Could you check a few things on this drawing? It's one solid part, dimensions in mm from its lowest x, y, z. Coordinates: 2 decimals unless noted, no trailing zeros. Order: outer loops, then holes, each group sorted by start corner. A loop starts at its lowest first (then second) coordinate and runs counter-clockwise, first axis right, second up.
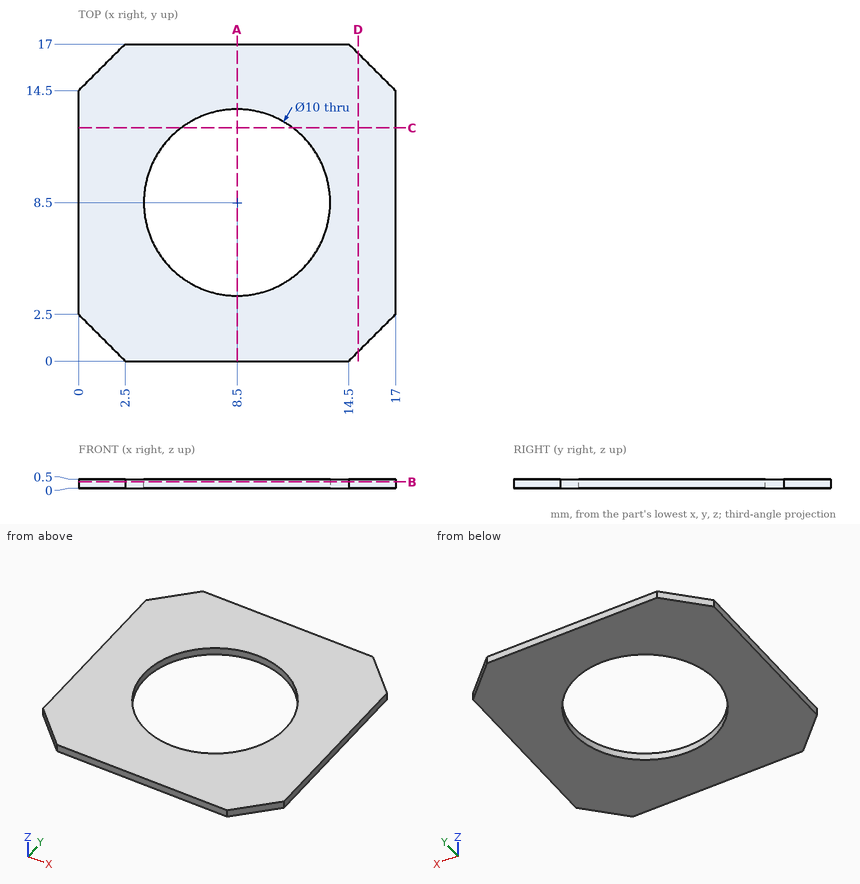
Item 1: I need wall thicknesses on line 1 (Y direction, x = 8.5, z = 0.3); line 2 (X direction, y = 7, z = 0.1); line 3 (Y direction, x = 12.75, z = 0.15). Which ranges of each line are inside material? Lowest first, please.
Item 2: Suppose I cut it at C-C (y = 12.5). List the corners of the cut face in (x, z) for me.
Item 3: Suppose I cut it at A-A (x = 8.5). List the corners of the cut face in (y, z) for me, and give its area (3 significant figures).
Item 4: Suppose I cut it at D-D (x = 15). List the corners of the cut face in (y, z) for me, and give its area (3 significant figures).
Item 5: For pin 1 Ø10 at (x, y) = (11.5, 8.5) entering from +Z, with a flat end and sliding along its axis, tell me the tip position at first contact or that it passes through.
Item 6: Suppose I cut it at B-B (z = 0.35). List the corners of the cut face in (x, y) for me, and give its area (3 significant figures).
Geometry results:
1. line 1: y = 0 to 3.5, 13.5 to 17
1. line 2: x = 0 to 3.73, 13.27 to 17
1. line 3: y = 0 to 5.87, 11.13 to 17
2. outline: (0, 0) - (5.5, 0) - (5.5, 0.5) - (0, 0.5) - close; (11.5, 0) - (17, 0) - (17, 0.5) - (11.5, 0.5) - close
3. outline: (0, 0) - (3.5, 0) - (3.5, 0.5) - (0, 0.5) - close; (13.5, 0) - (17, 0) - (17, 0.5) - (13.5, 0.5) - close
3. area: 3.50 mm2
4. outline: (0.5, 0) - (16.5, 0) - (16.5, 0.5) - (0.5, 0.5) - close
4. area: 8.00 mm2
5. pin 1: stops at z = 0.5
6. outline: (0, 2.5) - (2.5, 0) - (14.5, 0) - (17, 2.5) - (17, 14.5) - (14.5, 17) - (2.5, 17) - (0, 14.5) - close; hole circle Ø10 at (8.5, 8.5)
6. area: 198 mm2
